Verification items for this drawing (mm, ordinates from the low corner). A direction names the side the tool comes from. Round coordinates to 2 decimals unless told otherwise and drop trailing zeros. Order: outer loops, then holes, each group sorted by start corner. A loop starts at its lowest first (then second) coordinate and runs counter-clockwise, first axis right, second up. Notation, with made-up numbers: (-26.75, -24) -> (-8.75, -24) arc R14 cw to (-8.75, 2) -> close; hole circle Ø4 at (-13.5, 14.5). An arc over 180 degrees is marked (long way). Answer in a Markdown table with one row per item.
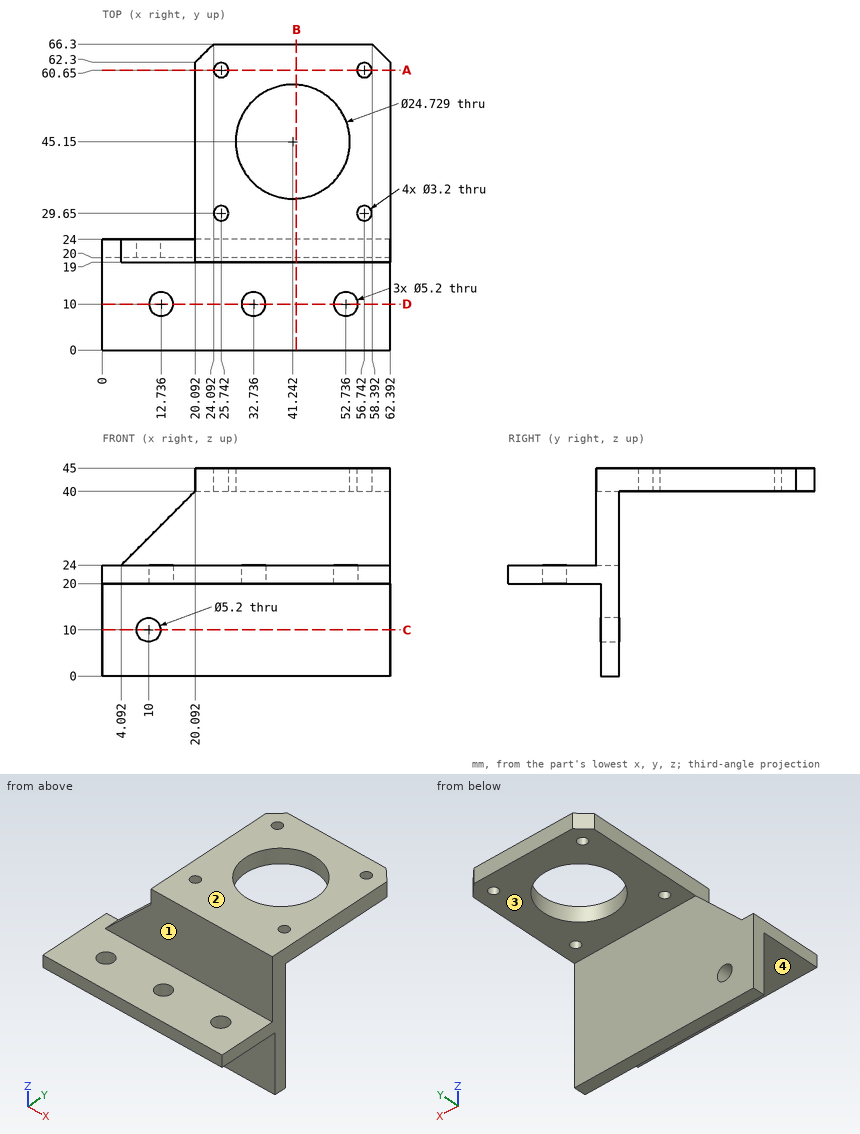
Item 1: Cross-section at B-B (x = 42). Record the boundary of the cut face in (y, z).
Result sheet:
| item | result |
|---|---|
| outline | (0, 20) -> (20, 20) -> (20, 0) -> (24, 0) -> (24, 40) -> (32.81, 40) -> (32.81, 45) -> (19, 45) -> (19, 24) -> (0, 24) -> close; (57.49, 40) -> (66.3, 40) -> (66.3, 45) -> (57.49, 45) -> close |
Item 2: Set-up check for the marked faces 1, 2, 3 and 4: record each of +Z, -Z, +X, -X, +Y, -Y from which the full face is reachable in a straight line by a thin tool's end or side.
Result sheet:
| item | result |
|---|---|
| face 1 | +Z, +X, -X, -Y |
| face 2 | +Z, +X, -X, +Y, -Y |
| face 3 | -Z, +X, -X, +Y |
| face 4 | -Z, +X, -X, -Y |
Item 3: Cross-section at A-A (y = 60.65). Record the boundary of the cut face in (x, z).
Result sheet:
| item | result |
|---|---|
| outline | (20.09, 40) -> (24.14, 40) -> (24.14, 45) -> (20.09, 45) -> close; (27.34, 40) -> (55.14, 40) -> (55.14, 45) -> (27.34, 45) -> close; (58.34, 40) -> (62.39, 40) -> (62.39, 45) -> (58.34, 45) -> close |
Item 4: Cross-section at C-C (z = 10). Record the boundary of the cut face in (x, y).
Result sheet:
| item | result |
|---|---|
| outline | (0, 20) -> (7.4, 20) -> (7.4, 24) -> (0, 24) -> close; (12.6, 20) -> (62.39, 20) -> (62.39, 24) -> (12.6, 24) -> close |
Item 5: Depth check by flat-ended pin: P1, Ø3, axis at x = 52.5, z = 29.5, coming from the -Y side; P2, Ø5, axis at x = 25.74, y = 29.65, coming from the -Z side; P3, Ø4, axis at x = 10, z = 10, coming from the +Y side; P4, Ø1, axis at x = 34.5, z = 27, coming from the +Y side. Enter the tip coordinate at first touch or a pass-through.
Result sheet:
| item | result |
|---|---|
| P1 | stops at y = 19 |
| P2 | stops at z = 40 |
| P3 | passes through |
| P4 | stops at y = 24 |
Item 6: Cross-section at D-D (y = 10). Record the boundary of the cut face in (x, z).
Result sheet:
| item | result |
|---|---|
| outline | (0, 20) -> (10.14, 20) -> (10.14, 24) -> (0, 24) -> close; (15.34, 20) -> (30.14, 20) -> (30.14, 24) -> (15.34, 24) -> close; (35.34, 20) -> (50.14, 20) -> (50.14, 24) -> (35.34, 24) -> close; (55.34, 20) -> (62.39, 20) -> (62.39, 24) -> (55.34, 24) -> close |
Item 7: Scan lines: line 1 (X direction, y = 60, z = 41) (1 decimal); line 2 (Z direction, x = 32, y = 55); line 3 (Z direction, x = 42, y = 6). Record each from-to range of solid material in increasing order. Write a range as [from, to].
Result sheet:
| item | result |
|---|---|
| line 1 | x = [20.1, 24.3], [27.2, 55.3], [58.2, 62.4] |
| line 2 | z = [40, 45] |
| line 3 | z = [20, 24] |
